Read the model definition and answer for the solid it produces. Units are mm, in the model's axes. A direction names the side the tool comes from. Coordinates: 2 decimals unless noted, no trailing zeros. Order: outer loops, then holes, each group sorted by start corner. A loop starts at its lowest first (then second) coordinate and runs counter-clockwise, first axis right, second up. Notation, with made-up numbers: (-4.5, -19) -> (34.5, -19) arc R27 cw to (34.5, 8) -> close; hole circle Ø3 at (-32, 4.25). An arc over 180 degrees is marked (long way). Answer as a JSON object with one key per item and string values. Group by question number.
1) Section C-C on y = 131 is taken. Determine the outline of the cut face in (x, z), and give its area (3 significant figures).
2) Consider L1, parallel to Y at x = -31.5, z = 10.5; L2, parallel to Y at x = -1, z = -14; L3, parallel to X at y = 135.5, z = 1.5. Determine where each line is inside the solid, lowest interval first.
3) Given pin 1 (22 mm diameter, centred on y = -14.5, z = 4.5, fed in from -X); pin 2 (6 mm diameter, centred on x = 29.5, z = 25, fed in from +Y); pin 3 (1 mm diameter, centred on y = -6, z = 17, fed in from -X), each flat-ended and moving along its own axis, determine where each tip first touches the part or whether it passes through.
4) Determine the mould class of faces 6 (the cylindrical face through (-10.953, -14.79, 14.284)), 7 (the flat face through (11.25, -25.5, -0.2)), 8 (the cylindrical face through (-0.28, -8.14, 2.25)) for opening direction Z: released by +Z, released by -Z, zero draft, split by the parting line, or undercut.
5) A tool of negligible diameter and unlimited length cuts with its end or side. For faces 1 (the flat face through (-11.25, -25.5, -0.2)), 2 (the flat face through (14, -26.546, 0)), 3 (the flat face through (-20, -12, 7)), 4 (the flat face through (20, -12, 7)), 5 (the cylindrical face through (15.686, -23.232, -6.085)), from which of +Z, -Z, +X, -X, +Y, -Y can it reach the whole face along a straight path? Write none if from no direction.
6) Section B-B on x = 0 is taken. Determine the outline of the cut face in (y, z).
7) Section D-D on x = 30 is taken. Determine the outline of the cut face in (y, z), and give its area (3 significant figures).
from build123d import *

# Parameters (mm, degrees)
SKETCH1_R               = 45
BOSS_EXTRUDE1_DEPTH     = 5
SKETCH2_R               = 10
BOSS_EXTRUDE2_DEPTH     = 140
SKETCH3_R               = 18
BOSS_EXTRUDE3_DEPTH     = 36
FILLET1_R               = 6
CUT_EXTRUDE1_DEPTH      = 159.350876221
CUT_EXTRUDE1_DEPTH_BACK = 159.350876221
SKETCH4_W               = 21.648814377
SKETCH4_H               = 22.5
SKETCH5_R               = 7.5
CUT_EXTRUDE2_DEPTH      = 162.907573943
SKETCH7_R               = 10
SKETCH7_R_2             = 7.5
BOSS_EXTRUDE4_DEPTH     = 20


with BuildPart() as part:
    # Sketch1 → Boss-Extrude1 (new body)
    with BuildSketch(Plane(origin=(0, 0, 0), x_dir=(1, 0, 0), z_dir=(0, 1, 0))):
        with Locations(Location((0, 0, 0), (0, 0, 270))):
            Circle(SKETCH1_R)
    extrude(amount=BOSS_EXTRUDE1_DEPTH)

    # Sketch2 → Boss-Extrude2 (add)
    with BuildSketch(Plane(origin=(0, 5, 0), x_dir=(1, 0, 0), z_dir=(0, 1, 0))):
        with Locations(Location((0, 0, 0), (0, 0, 270))):
            Circle(SKETCH2_R)
    extrude(amount=BOSS_EXTRUDE2_DEPTH)

    # Sketch3 → Boss-Extrude3 (add)
    with BuildSketch(Plane.XZ):
        with Locations(Location((0, 0, 0), (0, 0, 270))):
            Circle(SKETCH3_R)
    extrude(amount=BOSS_EXTRUDE3_DEPTH)

    # Fillet1
    fillet1_edges = [part.edges().sort_by_distance(p)[0] for p in [
        (0, -36, 18),
    ]]
    fillet(fillet1_edges, radius=FILLET1_R)

    # Sketch4 → Cut-Extrude1 (cut, two sides: drawn at the far end of the back side and taken through both)
    with BuildSketch(Plane.XY.offset(-CUT_EXTRUDE1_DEPTH_BACK)):
        with Locations((22.074407189, -15.296408269)):
            Rectangle(SKETCH4_W, SKETCH4_H)
        with Locations((-22.074407189, -15.296408269)):
            Rectangle(SKETCH4_W, SKETCH4_H)
    extrude(amount=CUT_EXTRUDE1_DEPTH + CUT_EXTRUDE1_DEPTH_BACK, mode=Mode.SUBTRACT)

    # Sketch5 → Cut-Extrude2 (cut, through all)
    with BuildSketch(Plane(origin=(11.25, 0, 0), x_dir=(0, 0, -1), z_dir=(1, 0, 0))):
        with Locations(Location((0, -15.296408269, 0), (0, 0, 90))):
            Circle(SKETCH5_R)
    extrude(amount=-CUT_EXTRUDE2_DEPTH, mode=Mode.SUBTRACT)

    # Sketch7 → Boss-Extrude4 (add, symmetric)
    with BuildSketch(Plane(origin=(0, 0, 0), x_dir=(0, 0, -1), z_dir=(1, 0, 0))):
        with Locations(Location((0, -15.296408269, 0), (0, 0, 90))):
            Circle(SKETCH7_R)
        with Locations(Location((0, -15.296408269, 0), (0, 0, 90))):
            Circle(SKETCH7_R_2, mode=Mode.SUBTRACT)
    extrude(amount=BOSS_EXTRUDE4_DEPTH, both=True)


solid = part.part
Worked answers:
{
 "1": {"outline": "circle Ø20 at (0, 0)", "area": "314 mm²"},
 "2": {"L1": "y = 0 to 5", "L2": "y = -35.64 to 5", "L3": "x = -9.89 to 9.89"},
 "3": {"pin 1": "stops at x = -20", "pin 2": "stops at y = 5", "pin 3": "stops at x = -7.19"},
 "4": {"face 6": "split by the parting line", "face 7": "zero draft", "face 8": "undercut"},
 "5": {"face 1": "-X", "face 2": "+Z, -Z, +X", "face 3": "+Z, -Z, -X, -Y", "face 4": "+Z, -Z, +X, -Y", "face 5": "+X"},
 "6": {"outline": "(-36, -12) arc R6 ccw to (-30, -18) -> (0, -18) -> (0, -45) -> (5, -45) -> (5, -10) -> (145, -10) -> (145, 10) -> (5, 10) -> (5, 45) -> (0, 45) -> (0, 18) -> (-30, 18) arc R6 ccw to (-36, 12) -> close; hole circle Ø15 at (-15.3, 0)"},
 "7": {"outline": "(0, -33.54) -> (5, -33.54) -> (5, 33.54) -> (0, 33.54) -> close", "area": "335 mm²"}
}
